Drawing for the job (mm, zero at the part's lowest x, y, z). A direction names the side the tool comes from. Coordinates: 2 decimals unless noted, no trailing zeros. Write each loop counter-clockwise with the first axis right and the second up, starting at its lowest first coordinate (ties: lowest second). Pieces come first, ordered by that corner, then holes. Notation, with made-up numbers: (-24, 84) -> (34, 84) arc R10 cw to (34, 90) -> close; hole circle Ø2 at (-29.75, -36.75). An arc over 180 degrees is marked (long way). Write item = value, one per line. Start each with the question number.
Q1. Band-saw the part on B-B, the plane x = 20. List the corners of the cut face in (y, z), plus the area to 3 significant figures.
Q2. Probe line 1 (Z direction, x = 20, y = 11.25); line 2 (Y direction, x = 15, z = 2.5); line 3 (Z direction, x = 20, y = 5.75). List the from-to ranges inside material, lowest first.
Q3. Band-saw the part on A-A, the plane z = 20. List the corners of the cut face in (x, y), plus the area to 3 significant figures.
Q4. Pull direction Y, two halves, no side cores. Call the marked faces 4, 5 and 6: released by +Y, released by -Y, zero draft, split by the parting line, or undercut.
Q5. Tool access for the marked faces 1, 2 and 3: list every direction of +Z, -Z, +X, -X, +Y, -Y with a clear straight run to the whole face (end or side of a thin tool).
Q6. Pin check, flat tips, straight feed: P1, Ø6, axis at y = 15.5, z = 8.5, coming from the -X side; P2, Ø5, axis at x = 20, z = 20, coming from the -Y side; P3, Ø5, axis at x = 9.5, y = 9.5, coming from the +Z side; P4, Ø8, axis at y = 2, z = 30, coming from the +X side. Stop position of each tip, or through.
Q7. Band-saw the part on D-D, the plane z = 26.5. List the corners of the cut face in (x, y).
Q8. Band-saw the part on C-C, the plane y = 4. List the corners of the cut face in (x, z).
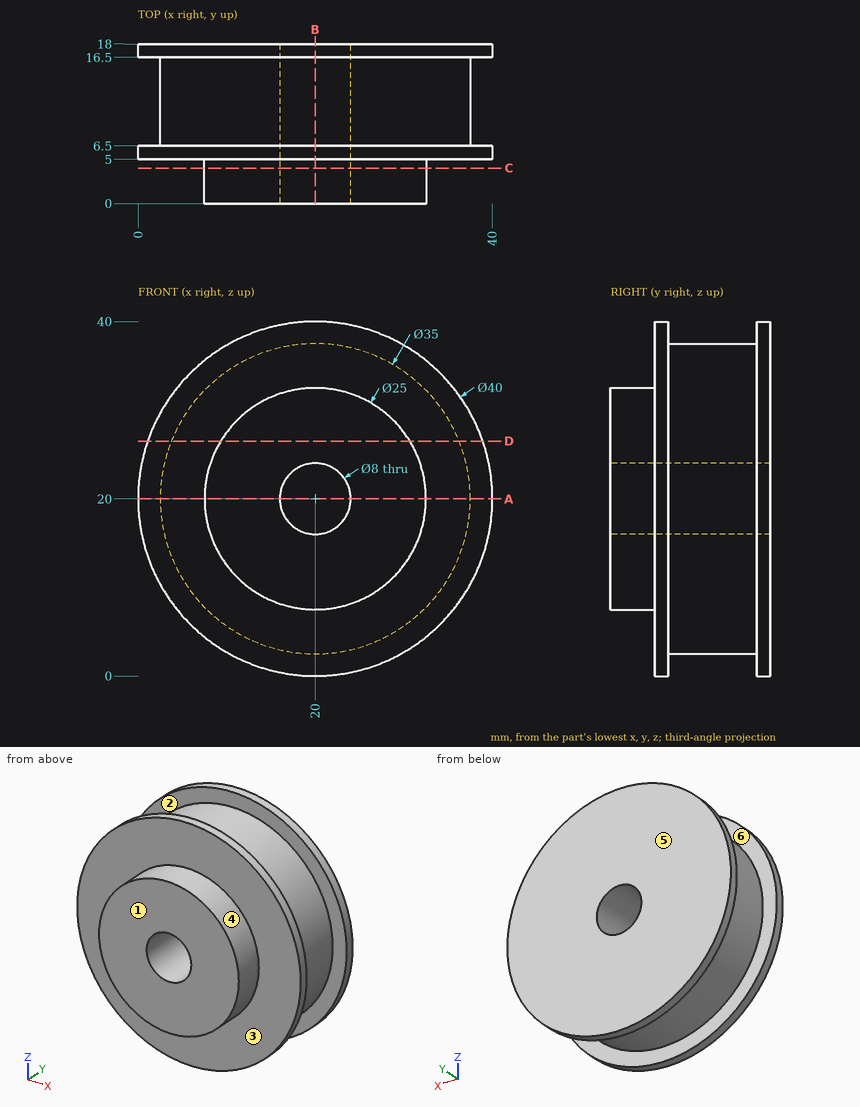
Ans:
q1.outline = (0, 7.5) -> (5, 7.5) -> (5, 0) -> (6.5, 0) -> (6.5, 2.5) -> (16.5, 2.5) -> (16.5, 0) -> (18, 0) -> (18, 16) -> (0, 16) -> close; (0, 24) -> (18, 24) -> (18, 40) -> (16.5, 40) -> (16.5, 37.5) -> (6.5, 37.5) -> (6.5, 40) -> (5, 40) -> (5, 32.5) -> (0, 32.5) -> close
q1.area = 451 mm2
q2.line_1 = 2.5 to 16, 24 to 37.5
q2.line_2 = 5 to 6.5, 16.5 to 18
q2.line_3 = 0 to 16, 24 to 40
q3.outline = (0, 5) -> (7.5, 5) -> (7.5, 0) -> (16, 0) -> (16, 18) -> (0, 18) -> (0, 16.5) -> (2.5, 16.5) -> (2.5, 6.5) -> (0, 6.5) -> close; (24, 0) -> (32.5, 0) -> (32.5, 5) -> (40, 5) -> (40, 6.5) -> (37.5, 6.5) -> (37.5, 16.5) -> (40, 16.5) -> (40, 18) -> (24, 18) -> close
q3.area = 451 mm2
q4.face_4 = zero draft
q4.face_5 = released by +Y
q4.face_6 = undercut
q5.face_1 = +Z, -Z, +X, -X, -Y
q5.face_2 = none
q5.face_3 = -Y
q6.P1 = 1.98
q6.P2 = through
q6.P3 = 35.56
q6.P4 = 38.6
q7.outline = (1.09, 5) -> (9.32, 5) -> (9.32, 0) -> (30.68, 0) -> (30.68, 5) -> (38.91, 5) -> (38.91, 6.5) -> (36.25, 6.5) -> (36.25, 16.5) -> (38.91, 16.5) -> (38.91, 18) -> (1.09, 18) -> (1.09, 16.5) -> (3.75, 16.5) -> (3.75, 6.5) -> (1.09, 6.5) -> close
q8.outline = circle Ø25 at (20, 20); hole circle Ø8 at (20, 20)
